from build123d import *

# Parameters (mm, degrees)
RESSALTO_EXTRUS_O1_DEPTH = 5
ESBO_O2_R                = 1.5
CORTE_EXTRUS_O1_DEPTH    = 5
ESBO_O4_R                = 0.5
ESBO_O4_W                = 12
ESBO_O4_H                = 23
CORTE_EXTRUS_O3_DEPTH    = 193.467750623
ESBO_O5_R                = 1.5
ESBO_O5_W                = 71.5
ESBO_O5_H                = 25
CORTE_EXTRUS_O4_DEPTH    = 193.467750623
ESBO_O6_R                = 6
CORTE_EXTRUS_O5_DEPTH    = 193.467750623


with BuildPart() as part:
    # Esboço1 → Ressalto-extrusão1 (new body)
    with BuildSketch(Plane(origin=(0, 0, 0), x_dir=(1, 0, 0), z_dir=(0, 1, 0))):
        with BuildLine():
            Line((-25.463589741, 142.264378701), (119.536410259, 142.264378701))
            ThreePointArc((119.536410259, 142.264378701), (126.607478071, 139.335446513), (129.536410259, 132.264378701))
            Line((129.536410259, 132.264378701), (129.536410259, -22.735621299))
            ThreePointArc((129.536410259, -22.735621299), (126.607478071, -29.806689111), (119.536410259, -32.735621299))
            Line((119.536410259, -32.735621299), (-25.463589741, -32.735621299))
            ThreePointArc((-25.463589741, -32.735621299), (-32.534657553, -29.806689111), (-35.463589741, -22.735621299))
            Line((-35.463589741, -22.735621299), (-35.463589741, 132.264378701))
            ThreePointArc((-35.463589741, 132.264378701), (-32.534657553, 139.335446513), (-25.463589741, 142.264378701))
        make_face()
    extrude(amount=RESSALTO_EXTRUS_O1_DEPTH)

    # Esboço2 → Corte-extrusão1 (cut)
    with BuildSketch(Plane(origin=(0, 5, 0), x_dir=(1, 0, 0), z_dir=(0, 1, 0))):
        with Locations(Location((-25.463589741, 7.264378701, 0), (0, 0, 270))):
            Circle(ESBO_O2_R)
        with Locations(Location((0.536410259, 126.264378701, 0), (0, 0, 270))):
            Circle(ESBO_O2_R)
        with Locations(Location((119.536410259, 102.264378701, 0), (0, 0, 270))):
            Circle(ESBO_O2_R)
        with Locations(Location((93.536410259, -16.735621299, 0), (0, 0, 270))):
            Circle(ESBO_O2_R)
    extrude(amount=-CORTE_EXTRUS_O1_DEPTH, mode=Mode.SUBTRACT)

    # Esboço4 → Corte-extrusão3 (cut, through all)
    with BuildSketch(Plane(origin=(0, 5, 0), x_dir=(1, 0, 0), z_dir=(0, 1, 0))):
        with Locations(Location((-9.463589741, 35.764378701, 0), (0, 0, 270))):
            Circle(ESBO_O4_R)
        with Locations(Location((-9.463589741, 63.764378701, 0), (0, 0, 270))):
            Circle(ESBO_O4_R)
        with Locations(Location((103.536410259, 45.764378701, 0), (0, 0, 270))):
            Circle(ESBO_O4_R)
        with Locations(Location((103.536410259, 73.764378701, 0), (0, 0, 270))):
            Circle(ESBO_O4_R)
        with Locations((-9.463589741, 49.764378701)):
            Rectangle(ESBO_O4_W, ESBO_O4_H)
        with Locations((103.536410259, 59.764378701)):
            Rectangle(ESBO_O4_W, ESBO_O4_H)
    extrude(amount=-CORTE_EXTRUS_O3_DEPTH, mode=Mode.SUBTRACT)

    # Esboço5 → Corte-extrusão4 (cut, through all)
    with BuildSketch(Plane(origin=(0, 5, 0), x_dir=(1, 0, 0), z_dir=(0, 1, 0))):
        with Locations(Location((-25.463589741, 89.264378701, 0), (0, 0, 270))):
            Circle(ESBO_O5_R)
        with Locations(Location((119.536410259, 20.264378701, 0), (0, 0, 270))):
            Circle(ESBO_O5_R)
        with Locations((47.036410259, 104.764378701)):
            Rectangle(ESBO_O5_W, ESBO_O5_H)
    extrude(amount=-CORTE_EXTRUS_O4_DEPTH, mode=Mode.SUBTRACT)

    # Esboço6 → Corte-extrusão5 (cut, through all)
    with BuildSketch(Plane(origin=(0, 5, 0), x_dir=(1, 0, 0), z_dir=(0, 1, 0))):
        with Locations(Location((-5.463589741, 112.264378701, 0), (0, 0, 270))):
            Circle(ESBO_O6_R)
        with Locations(Location((-5.463589741, 92.264378701, 0), (0, 0, 270))):
            Circle(ESBO_O6_R)
        with Locations(Location((99.536410259, 112.264378701, 0), (0, 0, 270))):
            Circle(ESBO_O6_R)
        with Locations(Location((99.536410259, 92.264378701, 0), (0, 0, 270))):
            Circle(ESBO_O6_R)
    extrude(amount=-CORTE_EXTRUS_O5_DEPTH, mode=Mode.SUBTRACT)


solid = part.part
Geometry: final body of the model. Coordinates: model frame, mm. A direction names the side the tool comes from. Give positions to 0.01 mm unless a question says otherwise; leave off trailing zeros. Write each loop counter-clockwise with the first axis right and the second up, starting at its lowest first coordinate (ties: lowest second). Pieces come first, ordered by that corner, then holes. Notation, with made-up numbers: (29.5, -29.5) -> (68.5, -29.5) arc R31 ccw to (68.5, 0.5) -> close; hole circle Ø2 at (43, 16.5). An arc over 180 degrees is marked (long way). Answer as a JSON object with one key per item and string values.
1. Cut plane B-B on z = -43. Output: boundary loops of the cut face in (x, y).
Ans:
{"outline": "(-35.46, 0) -> (-15.46, 0) -> (-15.46, 5) -> (-35.46, 5) -> close; (-3.46, 0) -> (129.54, 0) -> (129.54, 5) -> (-3.46, 5) -> close"}
2. Contact query for a flat-ended pin moving along its axis: pin 1 (1.8 mm diameter, centred on x = -25.46, z = -89.26, fed in from -Y). Output: stop coordinate, or through.
Ans:
{"pin 1": "passes through"}
3. Cut plane C-C on y = 4. Count the separate pieces of the cut face and the enclosed holes in it, and give its area (3 significant figures).
Ans:
{"separate pieces": "1", "enclosed holes": "17", "area": "26,000 mm^2"}
4. Cut plane A-A on x = 34.5. Output: boundary loops of the cut face in (y, z).
Ans:
{"outline": "(0, -142.26) -> (5, -142.26) -> (5, -117.26) -> (0, -117.26) -> close; (0, -92.26) -> (5, -92.26) -> (5, 32.74) -> (0, 32.74) -> close"}
5. Mould query, pull axis Z, two halves, no side actions, for faces 3 (the flat face through (-35.464, 2, -54)), 4 (the cylindrical face through (126.53, 2.46, -139.41)), 5 (the flat face through (97.536, 3, -60)), 6 (the cylindrical face through (-32.46, 2.46, 29.88)). Classes: pulls with the +Z half, pulls with the -Z half, needs draft (parallel to the pull), parting line crosses it, or undercut.
Ans:
{"face 3": "needs draft", "face 4": "pulls with the -Z half", "face 5": "undercut", "face 6": "pulls with the +Z half"}
6. Ray query, probe 1 along X at (y, z) = (1.65, -92); probe 2 along X at (y, z) = (0.3, -51); probe 3 along Z at (x, y) = (82, 3.4). Return the intervals inside material, ascending. Write a range as from..to.
Ans:
{"probe 1": "x = -35.46..-11.46, 0.53..93.54, 105.53..129.54", "probe 2": "x = -35.46..-15.46, -3.46..97.54, 109.54..129.54", "probe 3": "z = -142.26..-117.26, -92.26..32.74"}
7. Access query for faces 1 (the flat face through (48, 2, 32.736)), 2 (the flat face through (103, 3, -71.264)). Directions: +Z, -Z, +X, -X, +Y, -Y. A direction counts if a zero-diameter tool reaches every point of the face in a straight line with its end or side. Return the directions, or none.
Ans:
{"face 1": "+Z, +X, -X, +Y, -Y", "face 2": "+Y, -Y"}
